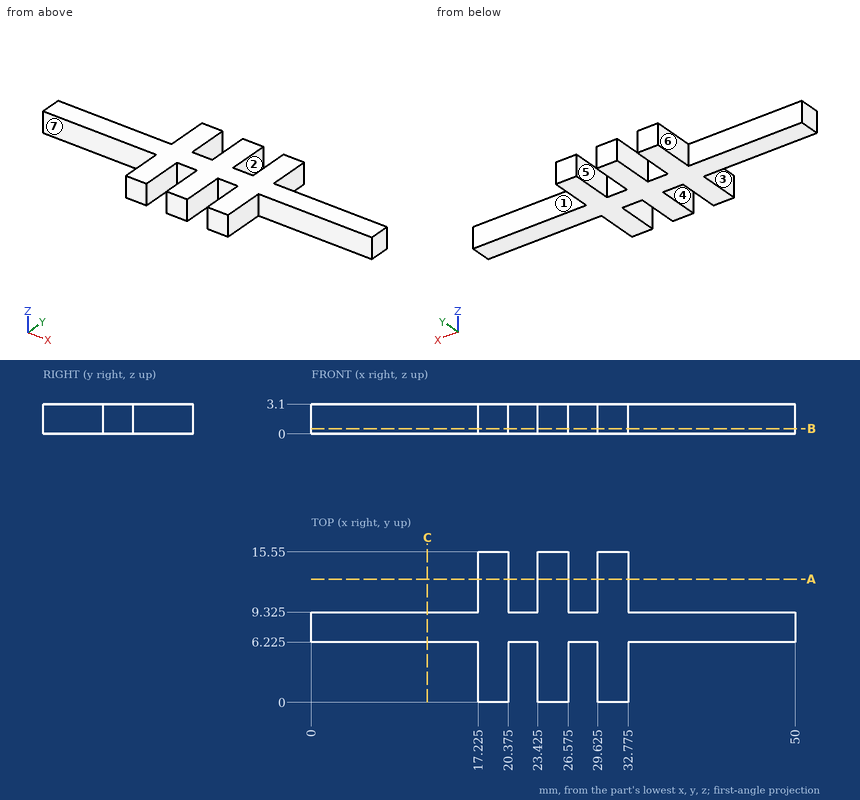
Design review of the part shown in the three views and the two pictorial views. Dimensions are in mm from the part's minimum x, y and z. A direction names the side the tool comes from. Round coordinates to 2 decimals unless told otherwise and drop trailing zeros. Loops run counter-clockwise (first coordinate to the right, second up) from the corner with the lowest first, then second, coordinate; pieces in that order, holes last. Notation, with made-up numbers: M 14.25,65 L 27.25,65 A12 ccw 27.25,76 Z; hole C 45.5,2.25 d3. An arc over 180 degrees is marked long. Write item = value, one per line.
Item 1: Insertion check: P1, Ø0.9, axis at y = 2.5, z = 1.5, coming from the -X side (3 decimals); P2, Ø1.5, axis at x = 21.5, z = 1, coming from the +Y side (3 decimals); P3, Ø1.5, axis at x = 21.5, z = 1, coming from the -Y side (3 decimals). Each pin has a flat end and moves straight along its axis. Give the tip position at first contact, or say it passes through.
Return value:
P1 = 17.225
P2 = 9.325
P3 = 6.225
Item 2: Take a section at B-B on z = 0.55. Write out the cut boundary in (x, y) (3 decimals).
Return value:
outline = M 0,6.225 L 17.225,6.225 L 17.225,0 L 20.375,0 L 20.375,6.225 L 23.425,6.225 L 23.425,0 L 26.575,0 L 26.575,6.225 L 29.625,6.225 L 29.625,0 L 32.775,0 L 32.775,6.225 L 50,6.225 L 50,9.325 L 32.775,9.325 L 32.775,15.55 L 29.625,15.55 L 29.625,9.325 L 26.575,9.325 L 26.575,15.55 L 23.425,15.55 L 23.425,9.325 L 20.375,9.325 L 20.375,15.55 L 17.225,15.55 L 17.225,9.325 L 0,9.325 Z
Item 3: Take a section at A-A on y = 12.75. Write out the cut boundary in (x, z) (3 decimals).
Return value:
outline = M 17.225,0 L 20.375,0 L 20.375,3.1 L 17.225,3.1 Z; M 23.425,0 L 26.575,0 L 26.575,3.1 L 23.425,3.1 Z; M 29.625,0 L 32.775,0 L 32.775,3.1 L 29.625,3.1 Z
Item 4: Machinability: for the marked faces 1, 2, 3 and 4, which of the approach directions +Z, -Z, +X, -X, +Y, -Y give a long, thin tool a straight path to every point of the face, cutting with its end or side? Answer none if there is none.
Return value:
face_1 = +Z, -Z, +X, +Y
face_2 = +Z, -Z, +Y
face_3 = +Z, -Z, -X, -Y
face_4 = +Z, -Z, -Y
Item 5: Take a section at C-C on x = 12. Write out the cut boundary in (y, z) (3 decimals), then the cut area to 3 significant figures.
Return value:
outline = M 6.225,0 L 9.325,0 L 9.325,3.1 L 6.225,3.1 Z
area = 9.61 mm2
Item 6: The part is to be moulded in two halves that separate along X. For the marked faces 5, 6 and 7, say which applies: released by +X, released by -X, zero draft, split by the parting line, or undercut.
Return value:
face_5 = undercut
face_6 = released by -X
face_7 = zero draft
Item 7: For line 1 (X direction, y = 12.75, z = 0.45) (3 decimals); line 2 (Y direction, x = 2, z = 1.65) (3 decimals), list the stretches that pass through material, from the lowest coordinate up. Write a range as [from, to].
Return value:
line_1 = [17.225, 20.375], [23.425, 26.575], [29.625, 32.775]
line_2 = [6.225, 9.325]
